Can you work these out from the drawing? Everything is in mm from the part's minimum corner. A direction names the side the tool comes from. Coordinates: 2 decimals unless noted, no trailing zeros.
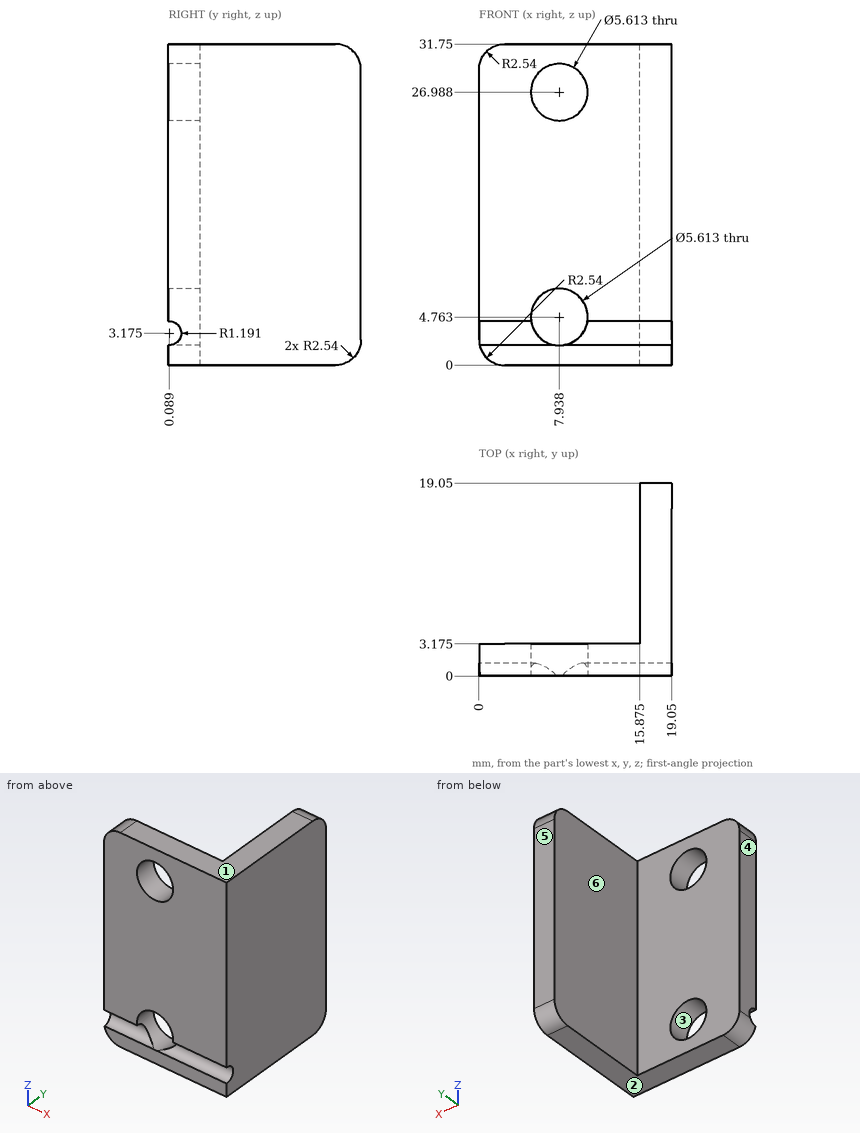
Item 1: We'd pull the mould along Z, two halves only. Please class the marked faces 1, 2, 3 and 4: +Z half, -Z half, draft (parallel to the pull), parting line (faces both ways), or undercut.
Results are:
face 1: +Z half
face 2: -Z half
face 3: undercut
face 4: draft
Item 2: I need wall thicknesses on line 1 along Y through (x, z) = (9, 9) (1 decimal); line 2 along Y through (x, z) = (15.25, 2.5) (1 decimal). Which ranges of each line are inside material? Lowest first, please.
Results are:
line 1: y = 0 to 3.2
line 2: y = 1.1 to 3.2
Item 3: I'm going to push flat-ended pins straight in: P1, Ø6, axis at x = 4, z = 15, coming from the +Y side (1 decimal); P2, Ø1, axis at y = 5, z = 26, coming from the -X side (1 decimal). Where does each tip first touch, or does it pass through?
Results are:
P1: stops at y = 3.2
P2: stops at x = 15.9
Item 4: On a 3-axis mill with a long thin cutter (end or side, diameter ignored), from which of +Z, -Z, +X, -X, +Y, -Y can I reach the whole of each face in a straight line? I mean the marked faces 5 and 6. Say none if no direction works.
Results are:
face 5: +Z, -Z, +X, -X, +Y
face 6: +Z, -Z, -X, +Y
